Could you check a few things on this model? Use its own coordinates, in mm. Face numbers are marked on the shaded views. A direction names the side the tool comes from. Give positions to 0.01 mm unless a question says otherwise; leave off trailing zeros. Loops run counter-clockwise (first coordinate to the right, second up) from the corner with the lowest first, then second, coordinate; pieces in that order, holes last. Notation, with made-up numbers: M -9,82.5 L 48,82.5 A31 ccw 48,114.5 Z; hole C -21,-0.75 d3. An arc over 180 degrees is marked long. Return JSON: item names as keys, results as strings. Group by question number.
1. For the marked faces 1, 2 and 3, which set-ups out of +Z, -Z, +X, -X, +Y, -Y let a thin tool reach every point of the face, with its end or its side?
2. If we section it at B-B (x = 0): Write out the boundary of the cut face in (y, z), plus the area to 3 significant figures.
3. If we section it at A-A (y = 0): Write out the boundary of the cut face in (x, z), plus the area to 3 significant figures.
4. Please list where these lines run through material, in increasing order: line 1 (Z direction, x = 5.5, y = 6); line 2 (Z direction, x = 1.5, y = 0); line 3 (X direction, y = -5.5, z = -39.5).
5. For pin 1 (1 mm diameter, centred on y = 8, z = -2.5, fed in from +X); pin 2 (12 mm diameter, centred on y = -7, z = -32.5, fed in from -X); pin 3 (2 mm diameter, centred on y = 12, z = -2.5, fed in from +X), each with a flat end and sliding along its axis, tell me the tip position at first contact or that it passes through.
6. If we section it at C-C (z = -35): Write out the boundary of the cut face in (x, y).
7. If we section it at D-D (y = 9): Write out the boundary of the cut face in (x, z), plus the area to 3 significant figures.
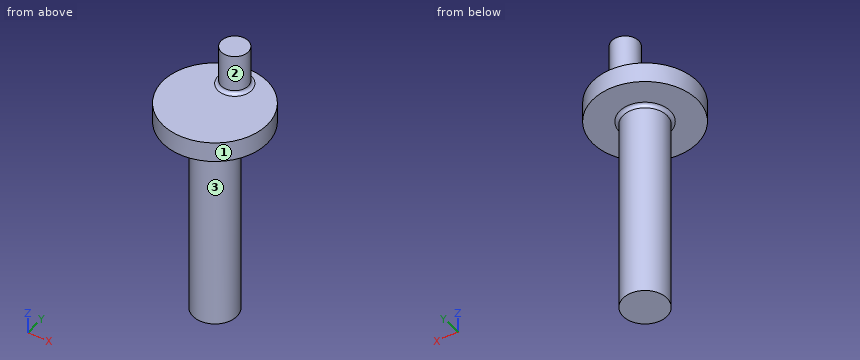
```python
from build123d import *

# Parameters (mm, degrees)
SKETCH1_R           = 15.5
BOSS_EXTRUDE2_DEPTH = 3
BOSS_EXTRUDE3_START = 3
SKETCH1_6_R         = 4
BOSS_EXTRUDE3_DEPTH = 12
SKETCH2_R           = 6.5
BOSS_EXTRUDE4_DEPTH = 60
FILLET1_R           = 1


with BuildPart() as part:
    # Sketch1 → Boss-Extrude2 (new, symmetric)
    with BuildSketch(Plane.XY):
        Circle(SKETCH1_R)
    extrude(amount=BOSS_EXTRUDE2_DEPTH, both=True)

    # Sketch1<6> → Boss-Extrude3 (add)
    with BuildSketch(Plane.XY.offset(BOSS_EXTRUDE3_START)):
        with Locations((0, 9)):
            Circle(SKETCH1_6_R)
    extrude(amount=BOSS_EXTRUDE3_DEPTH)

    # Sketch2 → Boss-Extrude4 (add)
    with BuildSketch(Plane(origin=(0, 0, -3), x_dir=(-1, 0, 0), z_dir=(0, 0, -1))):
        Circle(SKETCH2_R)
    extrude(amount=BOSS_EXTRUDE4_DEPTH)

    # Fillet1
    fillet1_edges = [part.edges().sort_by_distance(p)[0] for p in [
        (-4, 9, 3),
        (6.5, 0, -3),
    ]]
    fillet(fillet1_edges, radius=FILLET1_R)


solid = part.part
```
Answer:
{
 "1": {"face 1": "+Z, -Z", "face 2": "+Z", "face 3": "-Z"},
 "2": {"outline": "M -15.5,-3 L -7.5,-3 A1 cw -6.5,-4 L -6.5,-63 L 6.5,-63 L 6.5,-4 A1 cw 7.5,-3 L 15.5,-3 L 15.5,3 L 14,3 A1 cw 13,4 L 13,15 L 5,15 L 5,4 A1 cw 4,3 L -15.5,3 Z", "area": "1,060 mm²"},
 "3": {"outline": "M -15.5,-3 L -7.5,-3 A1 cw -6.5,-4 L -6.5,-63 L 6.5,-63 L 6.5,-4 A1 cw 7.5,-3 L 15.5,-3 L 15.5,3 L -15.5,3 Z", "area": "966 mm²"},
 "4": {"line 1": "z = -3 to 3", "line 2": "z = -63 to 3", "line 3": "x = -3.46 to 3.46"},
 "5": {"pin 1": "stops at x = 13.56", "pin 2": "stops at x = -6.42", "pin 3": "stops at x = 10.92"},
 "6": {"outline": "C 0,0 d13"},
 "7": {"outline": "M -12.62,-3 L 12.62,-3 L 12.62,3 L 5,3 A1 cw 4,4 L 4,15 L -4,15 L -4,4 A1 cw -5,3 L -12.62,3 Z", "area": "248 mm²"}
}
